Model file for the job. Use its own axes, mm. A direction names the side the tool comes from. Round coordinates to 2 decimals unless told otherwise and drop trailing zeros. Loops run counter-clockwise (first coordinate to the right, second up) from the corner with the lowest first, then second, coordinate; pieces in that order, holes last. Notation, with made-up numbers: M 45.25,-3 L 68.25,-3 A8 cw 68.25,5 Z; hole C -29,48 d4. An arc over 180 degrees is marked long. Use a Markdown table: item, result. Add a question column.
Item 1: Wall check: L1, parallel to Y at x = 42, z = 22; L2, parallel to Z at x = 7, y = -14; L3, parallel to X at y = -14, z = 16. Give the ranges that are in metal, low to high. Write a range as from..to.
Item 2: Saw through at B-B on y = -4.5. Write the cut outline in (x, z), then the cut area to 3 significant figures.
Item 3: Pin check, flat tips, straight feed: P1, Ø13.5, axis at x = 6.5, z = 22, coming from the -Y side; P2, Ø9.5, axis at x = 6.5, y = -23, coming from the +Z side; P3, Ø8.5, axis at y = -23, z = 25, coming from the -X side; P4, Ø5, axis at x = 44, y = -28.5, coming from the -Z side. Stop position of each tip, or through.
Item 4: Saw through at D-D on x = 27.5. Write the cut outline in (y, z).
Item 5: Tool access for faces 1 (the flat face through (31.75, -18, 17)), 2 (the flat face through (25, -16, 0)), 3 (the flat face through (19.05, -18, 17)): list every direction of +Z, -Z, +X, -X, +Y, -Y with a clear straight run to the whole face (end or side of a thin tool).
Item 6: Saw through at A-A on x = 15.5. Write the cut outline in (y, z).
Item 7: Saw through at C-C on z = 13.5. Write the cut outline in (x, y), then the cut area to 3 significant figures.
```python
from build123d import *

# Parameters (mm, degrees)
F1_DEPTH = 50.8
F3_DEPTH = 25.4
F4_W     = 12.7
F4_H     = 19.05
F5_DEPTH = 17.018
F7_DEPTH = 25.4


with BuildPart() as f1:
    # F0 (on Right) → F1 (new body)
    with BuildSketch(Plane.YZ):
        Polygon((-31.75, 12.7), (-31.75, 0), (0, 0), (0, 29.588299), (-12.7, 29.588299), (-12.7, 12.7), align=None)
    extrude(amount=F1_DEPTH)

    # F2 (on face) → F3 (cut)
    with BuildSketch(Plane.XZ.offset(12.7)):
        Polygon((38.373474, 29.588299), (50.8, 12.7), (50.8, 29.588299), align=None)
    extrude(amount=-F3_DEPTH, mode=Mode.SUBTRACT)

    # F4 (on face) → F5 (join)
    with BuildSketch(Plane.XY.offset(12.7)):
        with Locations((25.4, -22.225)):
            Rectangle(F4_W, F4_H)
    extrude(amount=F5_DEPTH)

    # F6 (on face) → F7 (cut)
    with BuildSketch(Plane.YZ.offset(31.75)):
        Polygon((-31.75, 29.718), (-31.75, 12.7), (-12.7, 29.588299), (-12.7, 29.718), align=None)
    extrude(amount=-F7_DEPTH, mode=Mode.SUBTRACT)


solid = f1.part
```
Entries:
| question | item | result |
|---|---|---|
| 1 | L1 | -12.7..0 |
| 1 | L2 | 0..12.7 |
| 1 | L3 | 19.05..31.75 |
| 2 | outline | M 0,0 L 50.8,0 L 50.8,12.7 L 38.37,29.59 L 0,29.59 Z |
| 2 | area | 1,400 mm2 |
| 3 | P1 | y = -12.7 |
| 3 | P2 | z = 12.7 |
| 3 | P3 | x = 19.05 |
| 3 | P4 | z = 0 |
| 4 | outline | M -31.75,0 L 0,0 L 0,29.59 L -12.7,29.59 L -31.75,12.7 Z |
| 5 | face 1 | +Z, +X, -Y |
| 5 | face 2 | -Z, +X, -X, +Y, -Y |
| 5 | face 3 | +Z, -X, -Y |
| 6 | outline | M -31.75,0 L 0,0 L 0,29.59 L -12.7,29.59 L -12.7,12.7 L -31.75,12.7 Z |
| 7 | outline | M 0,-12.7 L 19.05,-12.7 L 19.05,-30.85 L 31.75,-30.85 L 31.75,-12.7 L 50.21,-12.7 L 50.21,0 L 0,0 Z |
| 7 | area | 868 mm2 |
